The model under review builds one solid part; all positions refer to its coordinate system, in mm. Coordinates: 2 decimals unless noted, no trailing zeros. Write each loop counter-clockwise with the first axis right and the second up, starting at its lowest first coordinate (ties: lowest second). Pieces come first, ordered by that corner, then holes. Notation, with made-up numbers: (76, 64) - (101, 64) arc R30 cw to (101, 97) - close; hole circle Ø6 at (-14.75, 36). An arc over 180 degrees is marked (long way). Return JSON: item names as keys, results as strings. Group by question number.
(1) For pin 1 Ø6 at (x, y) = (-39.5, 31) entering from +Z; pin 2 Ø12 at (x, z) = (7.5, 9.5) entering from -Y; pin 3 Ø5 at (x, y) = (-8.5, 14.5) entering from -Z, all flat-tipped, find the tip position at first contact; note any pin that passes through.
(2) We need section A-A on x = -16.5. State the section outline as (y, z) points.
(3) We need section B-B on x = 22.5. State the section outline as (y, z) points.
(4) We need section C-C on x = -32. State the section outline as (y, z) points, then the cut area to 3 significant figures.
(5) To check wall thickness, follow L1, parallel to Z at x = -41, y = -8; L2, parallel to Y at x = 9, z = -24.5; L3, parallel to Z at x = -25, y = 17.5. State the ranges of each line that lie inside material, in increasing order. Write a range as from..to.
(6) Draft analysis for pull direction Y (two halves, no side actions). For faces 1 (the face through (-50.322, -37.804, -8.395)), 2 (the face through (34.921, 1, 1)), 3 (the face through (-22.6, 2.357, 7.486)), state which applies: released by +Y, released by -Y, zero draft, split by the parting line, or undercut.
```python
from build123d import *

# Parameters (mm, degrees)
F2_SIZE = 5
F3_SIZE = 5
F4_SIZE = 5


with BuildPart() as f1:
    # F0 (on Front) → F1 (revolve)
    with BuildSketch(Plane.XZ):
        Polygon((34.920584, 43.482468), (-50.5643, 43.482468), (-50.5643, 17.559418), (0, 0), (34.920584, 0), (34.920584, 17.559418), align=None)
    revolve(axis=Axis((17.460292, 0, 0), (-1, 0, 0)))

    # F2
    f2_edges = [f1.edges().sort_by_distance(p)[0] for p in [
        (-50.5643, 0, -43.482468),
    ]]
    chamfer(f2_edges, length=F2_SIZE)

    # F3
    f3_edges = [f1.edges().sort_by_distance(p)[0] for p in [
        (-50.5643, 0, -17.559418),
    ]]
    chamfer(f3_edges, length=F3_SIZE)

    # F4
    f4_edges = [f1.edges().sort_by_distance(p)[0] for p in [
        (34.920584, 0, -43.482468),
    ]]
    chamfer(f4_edges, length=F4_SIZE)


solid = f1.part
```
Ans:
{
 "1": {"pin 1": "z = 33.27", "pin 2": "y = -43.34", "pin 3": "z = -41.79"},
 "2": {"outline": "circle Ø86.96 at (0, 0); hole circle Ø11.46 at (0, 0)"},
 "3": {"outline": "circle Ø86.96 at (0, 0)"},
 "4": {"outline": "circle Ø86.96 at (0, 0); hole circle Ø22.23 at (0, 0)", "area": "5,550 mm²"},
 "5": {"L1": "-42.74..-11.78, 11.78..42.74", "L2": "-35.92..35.92", "L3": "-39.81..39.81"},
 "6": {"face 1": "split by the parting line", "face 2": "zero draft", "face 3": "undercut"}
}
